Build history of the part. All positions in model axes, mm. A direction names the side the tool comes from. Round coordinates to 2 decimals unless told otherwise and drop trailing zeros. Loops run counter-clockwise (first coordinate to the right, second up) from the corner with the lowest first, then second, coordinate; pieces in that order, holes last. Notation, with made-up numbers: (88.25, 34.25) - (135.25, 34.25) arc R25 ccw to (135.25, 65.25) - close; hole circle Ø3 at (15.25, 72.5). An arc over 180 degrees is marked (long way). Use one line per item in the form item = value. Start each with the question number.
Q1. Saw through at C-C (x = 16). Give the cut face in (y, z).
Q2. Saw through at B-B (z = 7.25). Give the cut face in (x, y).
Q3. Drill centre lines: line 1 (Y direction, x = -3, z = 8); line 2 (Y direction, x = 19.5, z = 17.5); line 3 (X direction, y = 10.5, z = 4.5). Where is each one in solid material? Low to high.
Q4. Saw through at A-A (x = -7). Give the cut face in (y, z), then the cut area to 3 significant figures.
Q5. Mould opens along Z. For faces 1 (the face through (21.49, 20.05, 3.26)), 2 (the face through (21.885, 20.054, 24.495)), 3 (the face through (11.219, 18.914, 12.878)) say: released by +Z, released by -Z, zero draft, split by the parting line, or undercut.
Q6. Saw through at D-D (y = 5). Give the cut face in (x, z), then the cut area to 3 significant figures.
Q7. 3-axis set-ups, long thin cutter, end or side, ignore diameter. For faces 4 (the face through (16, 19.187, 13)), 5 (the face through (-8.938, 0.843, 24.207)), 6 (the face through (-6, 1.709, 13)), 7 (the face through (22.755, 20.054, 3.904)): which of +Z, -Z, +X, -X, +Y, -Y reach the whole face in a straight line?
Q8. Pin check, flat tips, straight feed: pin 1 (6.5 mm diameter, centred on x = -7.5, z = 8, fed in from +Y); pin 2 (3.5 mm diameter, centred on x = -6.1, z = 3.97, fed in from +Y); pin 3 (5 mm diameter, centred on y = 11, z = 4, fed in from -X); pin 4 (10 mm diameter, centred on y = 15, z = 14.5, fed in from +X). Stop position of each tip, or through.
```python
from build123d import *

# Parameters (mm, degrees)
F1_DEPTH = 25.4
F2_R     = 1.8288
F3_DEPTH = 1.70942
F4_R     = 1.98374
F5_R     = 3.69316
F6_R     = 3.17499
F7_R     = 3.96875
F8_R     = 1.8288
F9_DEPTH = 1.70942


# Not quite as in the source:
# - a fillet or chamfer is up to 0.001 mm smaller than in the source, because OpenCascade refuses the exact size


with BuildPart() as f1:
    # F0 (on Top) → F1 (new body)
    with BuildSketch(Plane.XY):
        Polygon((-10.0697469202, 0), (0, 0), (11.077711991, 19.18716), (22.839589814, 19.18716), (22.839589814, 20.89658), (10.0907778938, 20.89658), (-0.9869340972, 1.70942), (-10.0697469202, 1.70942), align=None)
    extrude(amount=F1_DEPTH)

    # F2 (on face) → F3 (cut, through all)
    with BuildSketch(Plane(origin=(0, 20.89658, 0), x_dir=(-1, 0, 0), z_dir=(0, 1, 0))):
        with BuildLine():
            ThreePointArc((-22.839589814, 3.175), (-22.752350863, 3.914159458), (-22.4954281104, 4.6126993912))
            ThreePointArc((-22.4954281104, 4.6126993912), (-20.5594607088, 12.7), (-22.4954281104, 20.7873006088))
            ThreePointArc((-22.4954281104, 20.7873006088), (-22.752350863, 21.485840542), (-22.839589814, 22.225))
            Line((-22.839589814, 22.225), (-22.839589814, 3.175))
        make_face()
        with Locations((-19.664589814, 3.175)):
            Circle(F2_R)
        with Locations((-19.664589814, 22.225)):
            Circle(F2_R)
    extrude(amount=-F3_DEPTH, mode=Mode.SUBTRACT)

    # F4
    f4_edges = [f1.edges().sort_by_distance(p)[0] for p in [
        (-0.986934, 1.70942, 12.7),
        (11.077712, 19.18716, 12.7),
    ]]
    fillet(f4_edges, radius=F4_R)

    # F5
    f5_edges = [f1.edges().sort_by_distance(p)[0] for p in [
        (10.090778, 20.89658, 12.7),
        (0, 0, 12.7),
    ]]
    fillet(f5_edges, radius=F5_R)

    # F6 (radius 3.175 in the source; OpenCascade refuses exactly that, so slightly less here)
    f6_edges = [f1.edges().sort_by_distance(p)[0] for p in [
        (22.83959, 20.04187, 25.4),
        (22.83959, 20.04187, 0),
    ]]
    fillet(f6_edges, radius=F6_R)

    # F7
    f7_edges = [f1.edges().sort_by_distance(p)[0] for p in [
        (-10.069747, 0.85471, 25.4),
        (-10.069747, 0.85471, 0),
    ]]
    fillet(f7_edges, radius=F7_R)

    # F8 (on face) → F9 (cut, through all)
    with BuildSketch(Plane(origin=(0, 1.70942, 0), x_dir=(-1, 0, 0), z_dir=(0, 1, 0))):
        with Locations((6.1009969202, 3.96875)):
            Circle(F8_R)
        with Locations((6.1009969202, 21.43125)):
            Circle(F8_R)
    extrude(amount=-F9_DEPTH, mode=Mode.SUBTRACT)


solid = f1.part
```
Report:
q1.outline = (19.19, 0) - (20.9, 0) - (20.9, 25.4) - (19.19, 25.4) - close
q2.outline = (-10.07, 0) - (-2.13, 0) arc R3.69 ccw to (1.07, 1.85) - (10.51, 18.2) arc R1.98 cw to (12.22, 19.19) - (21.41, 19.19) - (21.41, 20.9) - (12.22, 20.9) arc R3.69 ccw to (9.02, 19.05) - (-0.41, 2.7) arc R1.98 cw to (-2.13, 1.71) - (-10.07, 1.71) - close
q3.line_1 = 0 to 1.71
q3.line_2 = 19.19 to 20.9
q3.line_3 = 4.09 to 6.06
q4.outline = (0, 0.1) - (1.71, 0.1) - (1.71, 2.38) - (0, 2.38) - close; (0, 5.56) - (1.71, 5.56) - (1.71, 19.84) - (0, 19.84) - close; (0, 23.02) - (1.71, 23.02) - (1.71, 25.3) - (0, 25.3) - close
q4.area = 32.2 mm²
q5.face_1 = undercut
q5.face_2 = released by +Z
q5.face_3 = zero draft
q6.outline = (0.91, 0) - (2.89, 0) - (2.89, 25.4) - (0.91, 25.4) - close
q6.area = 50.1 mm²
q7.face_4 = +Z, -Z, +X, -Y
q7.face_5 = +Z, -X, +Y, -Y
q7.face_6 = +Z, -Z, -X, +Y
q7.face_7 = +X, +Y, -Y
q8.pin_1 = 1.71
q8.pin_2 = through
q8.pin_3 = 2.93
q8.pin_4 = 21.14
